Design review of the part built by this model. Coordinates are the model's own, in mm. Face numbers are marked on the shaded views. Coordinates: 2 decimals unless noted, no trailing zeros. Loops run counter-clockwise (first coordinate to the right, second up) from the corner with the lowest first, then second, coordinate; pieces in that order, holes last. Notation, with made-up numbers: M 75,23 L 130,23 A17 ccw 130,48 Z; hole C 57.25,-11 d11. An arc over 180 degrees is marked long. One line per item, written item: value.
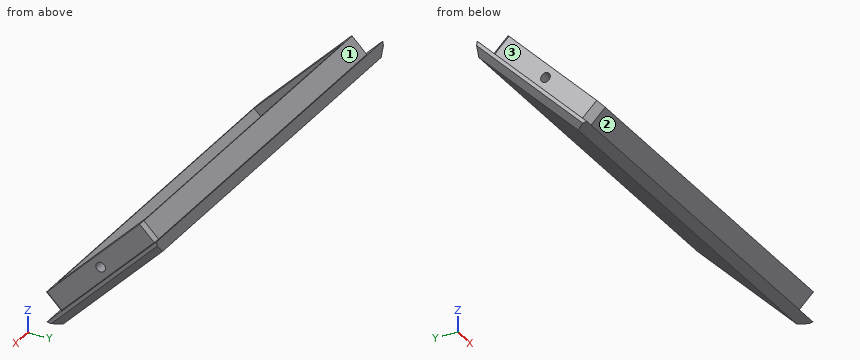
```python
from build123d import *

# Parameters (mm, degrees)
SKETCH018_W             = 120
SKETCH018_H             = 45
PAD003_DEPTH            = 3
SKETCH019_W             = 113.5
SKETCH019_H             = 40
PAD004_DEPTH            = 6
SKETCH020_R             = 1.4
POCKET008_DEPTH         = 116.751
POCKET012_DEPTH         = 376.9523572644
CHAMFER008_SIZE         = 2
SKETCH021_W             = 105
SKETCH021_H             = 37
POCKET013_DEPTH         = 6
CHAMFER009_SIZE         = 2
CHAMFER010_SIZE         = 1
CHAMFER011_SIZE         = 1
CHAMFER012_SIZE         = 2
BODY001_PLACEMENT_ANGLE = 45


with BuildPart() as part:
    # Sketch018 → Pad003 (new body)
    with BuildSketch(Plane.XZ):
        Rectangle(SKETCH018_W, SKETCH018_H)
    extrude(amount=PAD003_DEPTH)

    # Sketch019 (on Face6 of Pad003) → Pad004 (join)
    with BuildSketch(Plane.XZ.offset(3)):
        Rectangle(SKETCH019_W, SKETCH019_H)
    extrude(amount=PAD004_DEPTH)

    # Sketch020 (on Face8 of Pad004) → Pocket008 (cut, through all)
    with BuildSketch(Plane(origin=(56.75, 0, 0), x_dir=(0, 0, 1), z_dir=(1, 0, 0))):
        with Locations((0, 6)):
            Circle(SKETCH020_R)
    extrude(amount=-POCKET008_DEPTH, mode=Mode.SUBTRACT)

    # Sketch024 (on Face3 of Pocket008) → Pocket012 (cut, through all)
    with BuildSketch(Plane(origin=(60, 0, 0), x_dir=(0, 0, 1), z_dir=(1, 0, 0))):
        Polygon((-22.5, 3), (-17.8754562378, -3.604532956), (-35.516254, -3.604532956), align=None)
    pocket012 = extrude(amount=-POCKET012_DEPTH, mode=Mode.SUBTRACT)

    # Mirrored: Pocket012 across Sketch024 V_Axis
    add(pocket012.mirror(Plane(origin=(60, 0, 0), x_dir=(1, 0, 0), z_dir=(0, 0, 1))), mode=Mode.SUBTRACT)

    # Chamfer008
    chamfer008_edges = [part.edges().sort_by_distance(p)[0] for p in [
        (60, 0, 0),
        (-60, 0, 0),
    ]]
    chamfer(chamfer008_edges, length=CHAMFER008_SIZE)

    # Sketch021 → Pocket013 (cut)
    with BuildSketch(Plane.XZ.offset(9)):
        Rectangle(SKETCH021_W, SKETCH021_H)
    extrude(amount=-POCKET013_DEPTH, mode=Mode.SUBTRACT)

    # Chamfer009
    chamfer009_edges = [part.edges().sort_by_distance(p)[0] for p in [
        (-56.75, -6, -20),
    ]]
    chamfer(chamfer009_edges, length=CHAMFER009_SIZE)

    # Chamfer010
    chamfer010_edges = [part.edges().sort_by_distance(p)[0] for p in [
        (56.75, -6, -20),
    ]]
    chamfer(chamfer010_edges, length=CHAMFER010_SIZE)

    # Chamfer011
    chamfer011_edges = [part.edges().sort_by_distance(p)[0] for p in [
        (56.75, -6, 20),
    ]]
    chamfer(chamfer011_edges, length=CHAMFER011_SIZE)

    # Chamfer012
    chamfer012_edges = [part.edges().sort_by_distance(p)[0] for p in [
        (-56.75, -6, 20),
    ]]
    chamfer(chamfer012_edges, length=CHAMFER012_SIZE)


with BuildPart() as part_1:
    # Body001 placement: moved
    add(part.part.moved(Location((7, 18.7509559904, -18.0573149459))).rotate(Axis((7, 18.7509559904, -18.0573149459), (-1, 0, 0)), BODY001_PLACEMENT_ANGLE))


solid = part_1.part
```
(1) Mouldability with a two-part tool opening along Y and no side actions: class the marked faces 1, 2 and 3 as released by +Y, released by -Y, zero draft, split by the parting line, or undercut.
Reply:
face 1: undercut
face 2: released by -Y
face 3: zero draft
(2) To check wall thickness, follow line 1 along X through (y, z) = (11, -18); line 2 along Y through (x, z) = (-4, -27); line 3 along Z through (x, y) = (61.5, 14.5). State the ranges of each line that lie inside material, in increasing order. Write a range as [from, to].
Reply:
line 1: x = [-49.75, -45.5], [59.5, 63.75]
line 2: y = [-0.59, 1.53], [5.57, 9.81]
line 3: z = [-22.31, -15.21], [-12.41, -9.58]
(3) We need section A-A on x = 32. State the section outline as (y, z) points.
Reply:
outline: M -1.76,-25.84 L 2.49,-30.08 L 0.72,-31.85 L 4.33,-32.48 L 33.18,-3.63 L 32.54,-0.03 L 30.77,-1.79 L 26.53,2.45 L 25.47,1.39 L 29.71,-2.85 L 3.55,-29.02 L -0.69,-24.77 Z
(4) We need section B-B on z = -9. State the section outline as (x, y) points, then the cut area to 3 significant figures.
Reply:
outline: M -53,23.57 L -49.75,23.57 L -49.75,15.08 L -45.5,15.08 L -45.5,23.57 L 59.5,23.57 L 59.5,15.08 L 63.75,15.08 L 63.75,23.57 L 67,23.57 L 67,24.98 L 65,27.81 L -51,27.81 L -53,24.98 Z
area: 576 mm2
(5) Insertion check: pin 1 (9 mm diameter, centred on y = 9, z = -15.5, fed in from +X); pin 2 (6 mm diameter, centred on x = -40.5, z = -15.5, fed in from +Y); pin 3 (1.5 mm diameter, centred on x = 2, y = 27, fed in from -Z). Each pin has a flat end and moves straight along its axis. Give the tip position at first contact, or say it passes through.
Reply:
pin 1: stops at x = 63.75
pin 2: stops at y = 24.31
pin 3: stops at z = -10.56
(6) We need section C-C on y = 21.5. State the section outline as (x, z) points.
Reply:
outline: M -53,-12.48 L -51,-15.31 L 65,-15.31 L 67,-12.48 L 67,-11.07 L 63.75,-11.07 L 63.75,-2.58 L 59.5,-2.58 L 59.5,-11.07 L -45.5,-11.07 L -45.5,-2.58 L -49.75,-2.58 L -49.75,-11.07 L -53,-11.07 Z
